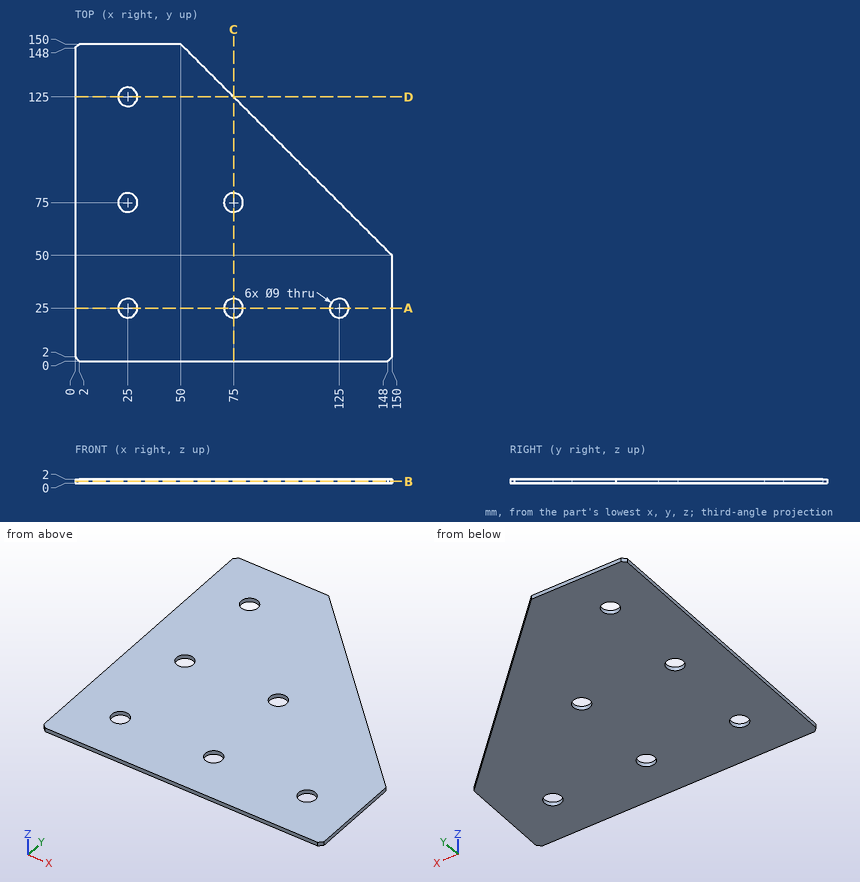
Verification items for this drawing (mm, ordinates from the low corner). Coordinates: 2 decimals unless noted, no trailing zeros. Loops run counter-clockwise (first coordinate to the right, second up) from the corner with the lowest first, then second, coordinate; pieces in that order, holes last.
Item 1: Sectioned sample at D-D, the plane y = 125. Record the boundary of the cut face in (x, z), then the cut area to 3 significant figures.
Item 2: Sectioned sample at B-B, the plane z = 0.85. Record the boundary of the cut face in (x, y).
Item 3: Sectioned sample at C-C, the plane x = 75. Record the boundary of the cut face in (y, z).
Item 4: Thickness scan on line 1 (Y direction, x = 25, z = 0.6); line 2 (X direction, y = 75, z = 1.15); line 3 (Y direction, x = 27, z = 0.2). Record the ranges inside material, lowest first.
Item 5: Sectioned sample at A-A, the plane y = 25. Record the boundary of the cut face in (x, z).
Check result:
1. outline: (0, 0) - (20.5, 0) - (20.5, 2) - (0, 2) - close; (29.5, 0) - (75, 0) - (75, 2) - (29.5, 2) - close
1. area: 132 mm2
2. outline: (0, 2) - (2, 0) - (148, 0) - (150, 2) - (150, 50) - (50, 150) - (2, 150) - (0, 148) - close; hole circle Ø9 at (25, 25); hole circle Ø9 at (25, 75); hole circle Ø9 at (25, 125); hole circle Ø9 at (75, 25); hole circle Ø9 at (75, 75); hole circle Ø9 at (125, 25)
3. outline: (0, 0) - (20.5, 0) - (20.5, 2) - (0, 2) - close; (29.5, 0) - (70.5, 0) - (70.5, 2) - (29.5, 2) - close; (79.5, 0) - (125, 0) - (125, 2) - (79.5, 2) - close
4. line 1: y = 0 to 20.5, 29.5 to 70.5, 79.5 to 120.5, 129.5 to 150
4. line 2: x = 0 to 20.5, 29.5 to 70.5, 79.5 to 125
4. line 3: y = 0 to 20.97, 29.03 to 70.97, 79.03 to 120.97, 129.03 to 150
5. outline: (0, 0) - (20.5, 0) - (20.5, 2) - (0, 2) - close; (29.5, 0) - (70.5, 0) - (70.5, 2) - (29.5, 2) - close; (79.5, 0) - (120.5, 0) - (120.5, 2) - (79.5, 2) - close; (129.5, 0) - (150, 0) - (150, 2) - (129.5, 2) - close
